Could you check a few things on this model? Use its own coordinates, in mm. Face numbers are marked on the shaded views. Coordinates: 2 decimals unless noted, no trailing zeros. Order: outer loops, then holes, each group sorted by start corner. A loop starts at its lowest first (then second) coordinate and runs counter-clockwise, first axis right, second up. Notation, with made-up numbers: (28, 13.25) -> (46, 13.25) arc R8 ccw to (46, 19.25) -> close; hole circle Ø2 at (69.5, 23.25). An arc over 180 degrees is marked (long way). Put each result on its own line as item: value. Start each with the question number.
Q1. If we section it at B-B (y = 64): Please give me the cut outline in (x, z), and give its area (3 significant figures).
Q2. We'd pull the mould along X, two halves only. Please class the marked faces 1, 2 and 3: +X half, -X half, draft (parallel to the pull), parting line (faces both ways), or undercut.
Q3. If we section it at A-A (x = -114): Please give me the cut outline in (y, z), and give its area (4 significant figures).
Q4. Please list where these lines run through material, in increasing order: line 1 along Y through (x, z) = (-53, 1.75); line 2 along Z through (x, y) = (-86.5, 84); line 3 along Z through (x, y) = (-61.5, 67).
Q5. If we section it at C-C (x = -78): Please give me the cut outline in (y, z), and give its area (3 significant figures).
Q6. Will these pins go through, and if not, where does the flat tip stop? pin 1 (16.5 mm diameter, centred on x = -105, y = 67.5, fed in from -Z); pin 2 (3 mm diameter, centred on x = -66.5, y = 63, fed in from -Z).
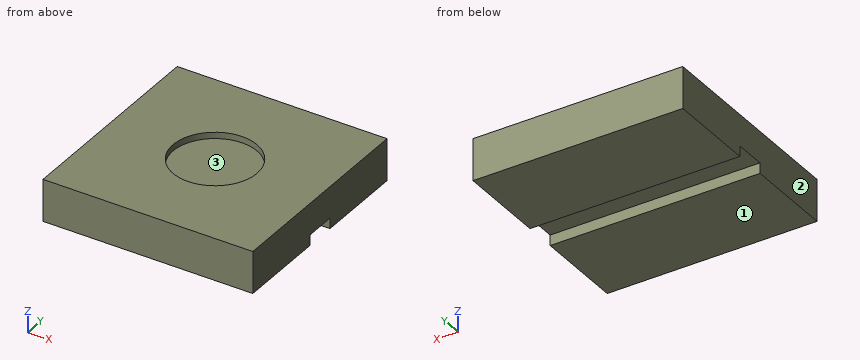
Solid Edge part; units mm, degrees
sketch "Sketch1" plane through (0, 0, 0) normal (0, 0, 1) x (1, 0, 0)
  line L0 (-141.1152, 15.9486) -> (-41.1152, 15.9486)
  line L1 (-41.1152, 15.9486) -> (-41.1152, 115.9486)
  line L2 (-41.1152, 115.9486) -> (-141.1152, 115.9486)
  line L3 (-141.1152, 115.9486) -> (-141.1152, 15.9486)
extrude "Protrusion1" add sketch "Sketch1" along normal blind 20
sketch "Sketch2" plane through (-66.1152, 40.9486, 20) normal (0, 0, 1) x (1, 0, 0)
  circle A0 centre (-25, 25) radius 20
  dimension "D1" = 25
extrude "ExtrudedCutout_1" cut sketch "Sketch2" against normal blind 3
sketch "Sketch3" plane through (-41.1152, 65.9486, 10) normal (1, 0, 0) x (0, 1, 0)
  line L0 (-7.5, -10) -> (7.5, -10)
  line L1 (7.5, -10) -> (7.5, -5)
  line L2 (7.5, -5) -> (-7.5, -5)
  line L3 (-7.5, -5) -> (-7.5, -10)
  dimension "D1" = 7.5
  dimension "D2" = 7.5
extrude "Cutout1" cut sketch "Sketch3" against normal through all
properties material "Aluminum, 6061-T6"
The answers:
1. outline: (-141.12, 5) -> (-41.12, 5) -> (-41.12, 20) -> (-71.21, 20) -> (-71.21, 17) -> (-111.02, 17) -> (-111.02, 20) -> (-141.12, 20) -> close
1. area: 1,380 mm^2
2. face 1: draft
2. face 2: -X half
2. face 3: undercut
3. outline: (15.95, 0) -> (58.45, 0) -> (58.45, 5) -> (73.45, 5) -> (73.45, 0) -> (115.95, 0) -> (115.95, 20) -> (15.95, 20) -> close
3. area: 1,925 mm^2
4. line 1: 15.95 to 58.45, 73.45 to 115.95
4. line 2: 0 to 17
4. line 3: 5 to 20
5. outline: (15.95, 0) -> (58.45, 0) -> (58.45, 5) -> (73.45, 5) -> (73.45, 0) -> (115.95, 0) -> (115.95, 20) -> (81.05, 20) -> (81.05, 17) -> (50.85, 17) -> (50.85, 20) -> (15.95, 20) -> close
5. area: 1,830 mm^2
6. pin 1: z = 0
6. pin 2: z = 5
